from build123d import *

# Parameters (mm, degrees)
SKETCH_1_R          = 10
EXTRUDE_1_DEPTH     = 4
SKETCH_2_R          = 2.5
CUT_EXTRUDE_1_DEPTH = 4
CUT_EXTRUDE_1_DRAFT = 39
FILLET_2_R          = 0.5
FILLET_3_R          = 0.5


with BuildPart() as part:
    # 草图1 → 凸台-拉伸1 (new body)
    with BuildSketch(Plane(origin=(0, 0, 0), x_dir=(1, 0, 0), z_dir=(0, 1, 0))):
        with Locations(Location((0, 0, 0), (0, 0, 270))):
            Circle(SKETCH_1_R)
    extrude(amount=EXTRUDE_1_DEPTH)


with BuildPart() as cut_extrude_1_tool:
    # 草图2 → 切除-拉伸1 (with draft: the straight prism first)
    with BuildSketch(Plane(origin=(0, 4, 0), x_dir=(1, 0, 0), z_dir=(0, 1, 0))):
        Circle(SKETCH_2_R)
    extrude(amount=-CUT_EXTRUDE_1_DEPTH)
    # 切除-拉伸1: the draft: its side faces are tilted about the plane it starts from
    cut_extrude_1_sides = [cut_extrude_1_tool.faces().sort_by_distance(p)[0] for p in [
        (-2.5, 2, 0),
    ]]
    draft(cut_extrude_1_sides, Plane(origin=(0, 4, 0), x_dir=(1, 0, 0), z_dir=(0, 1, 0)), CUT_EXTRUDE_1_DRAFT)


with BuildPart() as part_1:
    add(part.part)

    # 切除-拉伸1: cut by cut_extrude_1_tool
    add(cut_extrude_1_tool.part, mode=Mode.SUBTRACT)

    # 圆角2
    fillet_2_edges = [part_1.edges().sort_by_distance(p)[0] for p in [
        (0, 0, -10),
    ]]
    fillet(fillet_2_edges, radius=FILLET_2_R)

    # 圆角3
    fillet_3_edges = [part_1.edges().sort_by_distance(p)[0] for p in [
        (0, 4, -10),
    ]]
    fillet(fillet_3_edges, radius=FILLET_3_R)


solid = part_1.part
Geometry check sheet. Reference: the model listing, model coordinates, mm. Give positions to 0.01 mm unless a question says otherwise; leave off trailing zeros. Loops run counter-clockwise (first coordinate to the right, second up) from the corner with the lowest first, then second, coordinate; pieces in that order, holes last.
(1) Section check D-D on y = 3.75. Record the cut outline in (x, z), then the cut area to 3 significant figures.
From the geometry:
outline: circle Ø19.87 at (0, 0); hole circle Ø5.4 at (0, 0)
area: 287 mm2
(2) Release check for a two-part mould opening along Z. For faces 1 (the flat face through (-2, 4, 2)), 2 (the conical face through (2.53, 3.81, -0.8)), 3 (the cylindrical face through (-9.76, 1.98, -2.17)) record: released by +Z, released by -Z, zero draft, split by the parting line, or undercut.
From the geometry:
face 1: zero draft
face 2: undercut
face 3: split by the parting line
(3) Depth check by flat-ended pin: pin 1 Ø1.5 at (y, z) = (2.5, 2.5) entering from +X; pin 2 Ø10 at (x, z) = (-4, -1) entering from -Y; pin 3 Ø1 at (x, y) = (-6, 2) entering from +Z. Enter the tip coordinate at first touch or a pass-through.
From the geometry:
pin 1: stops at x = 9.85
pin 2: stops at y = 0
pin 3: stops at z = 8.35
(4) Thickness scan on L1, parallel to Z at x = 4, y = 1; L2, parallel to X at y = 2.5, z = 3; L3, parallel to X at y = 2.2, z = 3. Record the ranges inside material, lowest first.
From the geometry:
L1: z = -9.17 to -2.88, 2.88 to 9.17
L2: x = -9.54 to -2.19, 2.19 to 9.54
L3: x = -9.54 to -2.58, 2.58 to 9.54
(5) Section check A-A on z = 0. Record the cut outline in (x, y), then the cut area to 3 significant figures.
From the geometry:
outline: (-10, 0.5) arc R0.5 ccw to (-9.5, 0) - (-5.74, 0) - (-2.5, 4) - (-9.5, 4) arc R0.5 ccw to (-10, 3.5) - close; (2.5, 4) - (5.74, 0) - (9.5, 0) arc R0.5 ccw to (10, 0.5) - (10, 3.5) arc R0.5 ccw to (9.5, 4) - close
area: 46.8 mm2
(6) Section check B-B on x = 0. Record the cut outline in (y, z).
From the geometry:
outline: (0, -9.5) arc R0.5 ccw to (0.5, -10) - (3.5, -10) arc R0.5 ccw to (4, -9.5) - (4, -2.5) - (0, -5.74) - close; (0, 5.74) - (4, 2.5) - (4, 9.5) arc R0.5 ccw to (3.5, 10) - (0.5, 10) arc R0.5 ccw to (0, 9.5) - close
(7) Section check C-C on y = 1.9. Record the cut outline in (x, z).
From the geometry:
outline: circle Ø20 at (0, 0); hole circle Ø8.4 at (0, 0)
